```python
from build123d import *

# Parameters (mm, degrees)
F1_DEPTH = 100
F2_R     = 61.269346
F3_DEPTH = 97
F4_R     = 5
F5_DEPTH = 25


with BuildPart() as f1:
    # F0 (on Top) → F1 (new body)
    with BuildSketch(Plane.XY):
        Polygon((6.523423, 65.423498), (-20.813363, 62.254017), (-44.497616, 48.239678), (-60.434112, 25.80369), (-65.867287, -1.174563), (-59.857696, -28.030294), (-43.444451, -50.119905), (-19.465552, -63.6239), (7.932832, -66.207316), (34.013272, -57.423458), (54.266222, -38.791133), (65.189763, -13.532041), (64.895117, 13.986292), (53.433229, 39.005697), (32.785965, 57.200091), align=None)
    extrude(amount=F1_DEPTH)

    # F2 (on face) → F3 (cut)
    with BuildSketch(Plane.XY.offset(100)):
        Circle(F2_R)
    extrude(amount=-F3_DEPTH, mode=Mode.SUBTRACT)

    # F4 (on face) → F5 (cut)
    with BuildSketch(Plane.XY.offset(3)):
        Circle(F4_R)
    extrude(amount=-F5_DEPTH, mode=Mode.SUBTRACT)


solid = f1.part
```
Read the model definition and answer for the solid it produces. Units are mm, in the model's axes. A direction names the side the tool comes from. Give positions to 0.01 mm unless a question says otherwise; leave off trailing zeros. Write each loop counter-clockwise with the first axis right and the second up, starting at its lowest first coordinate (ties: lowest second). Pieces come first, ordered by that corner, then holes. Notation, with made-up numbers: (44.5, 70) - (66.5, 70) arc R10 cw to (66.5, 79) - close; hole circle Ø8 at (9.25, -0.5). An arc over 180 degrees is marked (long way). Write item = value, one per line. Start each with the question number.
Item 1: Find section B-B (x = 0). Give the vertices of the cut face in (y, z).
Item 2: Find section C-C (y = -43). Give the vertices of the cut face in (x, z), then the cut area to 3 significant figures.
Item 3: The mould has two halves that part along X. Classify faces 1 (the flat face through (59.244, 26.321, 49.3)), 2 (the flat face through (13, 1, 3)), 3 (the flat face through (-5.958, -64.898, 49.3)): +X half, -X half, draft (parallel to the pull), parting line (faces both ways), or undercut.
Item 4: Find the intervals of material crossed by probe 1 along Z at (x, y) = (9.5, 16); probe 2 along Y at (x, z) = (-47.5, 89); probe 3 along Y at (x, z) = (-6.5, 6.5), in increasing order. Write a range as [from, to].
Item 5: Find section A-A (z = 86). Give the vertices of the cut face in (x, y), then the cut area to 3 significant figures.
Item 6: A tool of negligible diameter and unlimited length cuts with its end or side. For faces 4 (the flat face through (13, 1, 0)), 5 (the cylindrical face through (-13.282, -59.812, 52.179)), from which of +Z, -Z, +X, -X, +Y, -Y can it reach the whole face along a straight path? Write none if from no direction.
Item 7: Each of these flat-tipped pins is pushed along its axis until it touches: P1, Ø5, axis at x = -36, z = 70.5, coming from the -Y side; P2, Ø3, axis at x = -9.5, z = 88.5, coming from the -Y side (3 decimals); P3, Ø1, axis at y = 23.5, z = 24, coming from the -X side. Where does it stop, or does it pass through?
Item 8: Find section D-D (x = 45). Give the vertices of the cut face in (y, z).
Response:
q1.outline = (-65.46, 0) - (-5, 0) - (-5, 3) - (-61.27, 3) - (-61.27, 100) - (-65.46, 100) - close; (5, 0) - (64.67, 0) - (64.67, 100) - (61.27, 100) - (61.27, 3) - (5, 3) - close
q2.outline = (-48.73, 0) - (49.69, 0) - (49.69, 100) - (43.65, 100) - (43.65, 3) - (-43.65, 3) - (-43.65, 100) - (-48.73, 100) - close
q2.area = 1,380 mm²
q3.face_1 = +X half
q3.face_2 = undercut
q3.face_3 = -X half
q4.probe_1 = [0, 3]
q4.probe_2 = [-44.66, -38.7], [38.7, 44.01]
q4.probe_3 = [-64.85, -60.92], [60.92, 63.91]
q5.outline = (-65.87, -1.17) - (-59.86, -28.03) - (-43.44, -50.12) - (-19.47, -63.62) - (7.93, -66.21) - (34.01, -57.42) - (54.27, -38.79) - (65.19, -13.53) - (64.9, 13.99) - (53.43, 39.01) - (32.79, 57.2) - (6.52, 65.42) - (-20.81, 62.25) - (-44.5, 48.24) - (-60.43, 25.8) - close; hole circle Ø122.54 at (0, 0)
q5.area = 1,570 mm²
q6.face_4 = -Z, +X, -X, +Y, -Y
q6.face_5 = +Z
q7.P1 = -55.72
q7.P2 = -64.705
q7.P3 = -61
q8.outline = (-47.32, 0) - (46.44, 0) - (46.44, 100) - (41.58, 100) - (41.58, 3) - (-41.58, 3) - (-41.58, 100) - (-47.32, 100) - close
